Could you check a few things on this model? Use its own coordinates, in mm. Face numbers are marked on the shaded views. A direction names the side the tool comes from. Coordinates: 2 decimals unless noted, no trailing zeros. Loops run counter-clockwise (first coordinate to the right, second up) from the corner with the lowest first, then second, coordinate; pieces in that order, holes last. Notation, with made-up numbers: (32, 87) - (63, 87) arc R19 ccw to (63, 103) - close; hole circle Ø10 at (57, 64). An arc over 180 degrees is marked (long way). One line per item, written item: value. Start each with the question number.
(1) If we section it at C-C on y = -54.5: Write out the boundary of the cut face in (x, z).
(2) If I drill on line 1 along Z through (x, y) = (24, -58.5); line 2 along X through (y, z) = (-29, 18) (3 decimals); line 3 along X through (y, z) = (-68, 5), over which ranges is the centre line in solid material (lowest first)? Write a range as from..to.
(3) If we section it at D-D on x = 10: Write out the boundary of the cut face in (y, z).
(4) If we section it at B-B on z = 10: Write out the boundary of the cut face in (x, y).
(5) If we section it at A-A on x = 0: Write out the boundary of the cut face in (y, z).
(6) If we mould it in two halves opening along Z, with no side actions, what happens to the marked faces 4, 5 and 6? For each: pulls with the +Z half, pulls with the -Z half, needs draft (parallel to the pull), parting line crosses it, or undercut.
(7) On a 3-axis mill with a long thin cutter (end or side, diameter ignored), from which of +Z, -Z, +X, -X, +Y, -Y can I reach the whole of each face in a straight line? I mean the marked faces 1, 2 and 3. Say none if no direction works.
(8) I'm going to push flat-ended pins straight in: P1, Ø6, axis at x = -22, y = -14, coming from the +Z side; P2, Ø9.5, axis at x = 1, y = -11, coming from the +Z side. Where does each tip first touch, or does it pass through?
```python
from build123d import *

# Parameters (mm, degrees)
F0_W     = 71.2816417217
F0_H     = 40.4414199293
F2_DEPTH = 101.6
F1_W     = 49.7516710311
F1_H     = 12.2197093442
F3_DEPTH = 101.6
F4_R     = 4.4126696885
F5_DEPTH = 6.35
F6_W     = 55.8680891991
F6_H     = 44.7704729486
F7_DEPTH = 101.6
F8_DEPTH = 6.35


with BuildPart() as f2:
    # F0 (on Front) → F2 (new body)
    with BuildSketch(Plane.XZ):
        with Locations((-1.6001984477, -0.1454725862)):
            Rectangle(F0_W, F0_H)
    extrude(amount=F2_DEPTH)

    # F1 (on Front) → F3 (cut)
    with BuildSketch(Plane.XZ):
        with Locations((-0.4364186898, 6.1098546721)):
            Rectangle(F1_W, F1_H)
    extrude(amount=F3_DEPTH, mode=Mode.SUBTRACT)

    # F4 (on Top) → F5 (join)
    with BuildSketch(Plane.XY):
        with Locations((0, -9.3056354672)):
            Circle(F4_R)
    extrude(amount=F5_DEPTH)

    # F6 (on Top) → F7 (cut)
    with BuildSketch(Plane.XY):
        with Locations((-4.929035902, -22.1368068433)):
            Rectangle(F6_W, F6_H)
    extrude(amount=F7_DEPTH, mode=Mode.SUBTRACT)

    # F4 (on Top) → F8 (join)
    with BuildSketch(Plane.XY):
        with Locations((0, -9.3056354672)):
            Circle(F4_R)
    extrude(amount=F8_DEPTH)


solid = f2.part
```
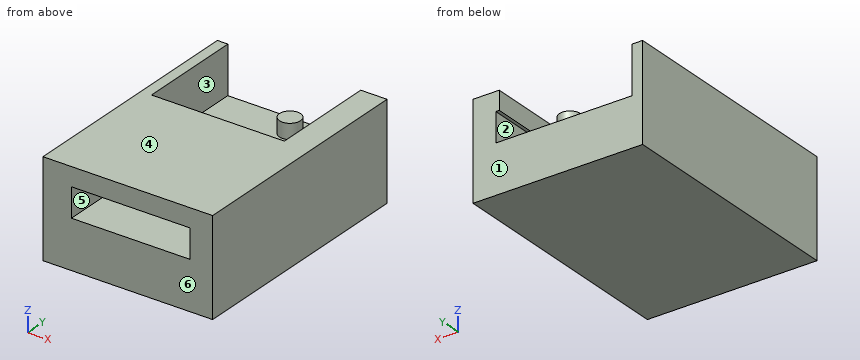
Values:
1. outline: (-37.24, -20.37) - (34.04, -20.37) - (34.04, 20.08) - (-37.24, 20.08) - close; hole (-25.31, 0) - (24.44, 0) - (24.44, 12.22) - (-25.31, 12.22) - close
2. line 1: z = -20.37..0, 12.22..20.08
2. line 2: x = -37.241..-32.863, 23.005..34.041
2. line 3: x = -37.24..-25.31, 24.44..34.04
3. outline: (-101.6, -20.37) - (0, -20.37) - (0, 0) - (-101.6, 0) - close; (-101.6, 12.22) - (-44.52, 12.22) - (-44.52, 20.08) - (-101.6, 20.08) - close
4. outline: (-37.24, -101.6) - (-25.31, -101.6) - (-25.31, -44.52) - (-32.86, -44.52) - (-32.86, 0) - (-37.24, 0) - close; (24.44, -101.6) - (34.04, -101.6) - (34.04, 0) - (24.44, 0) - close
5. outline: (-101.6, -20.37) - (0, -20.37) - (0, 0) - (-4.89, 0) - (-4.89, 6.35) - (-13.72, 6.35) - (-13.72, 0) - (-101.6, 0) - close; (-101.6, 12.22) - (-44.52, 12.22) - (-44.52, 20.08) - (-101.6, 20.08) - close
6. face 4: pulls with the +Z half
6. face 5: undercut
6. face 6: needs draft
7. face 1: +Z, -Z, +X, -X, +Y
7. face 2: +Y, -Y
7. face 3: +Z, +Y
8. P1: stops at z = 0
8. P2: stops at z = 6.35
